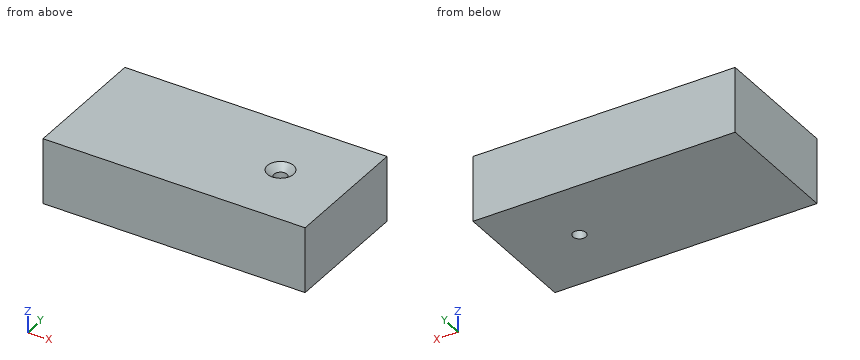
from build123d import *

# Parameters (mm, degrees)
F0_W           = 200
F0_H           = 100
F1_DEPTH       = 50
F3_D           = 10
F3_CSINK_D     = 20
F3_CSINK_ANGLE = 90


with BuildPart() as f1:
    # F0 (on Top) → F1 (new body)
    with BuildSketch(Plane.XY):
        with Locations((100, 50)):
            Rectangle(F0_W, F0_H)
    extrude(amount=F1_DEPTH)

    # F3 (through all)
    with Locations(Plane.XY.offset(50)):
        with Locations((150, 50)):
            CounterSinkHole(F3_D / 2, F3_CSINK_D / 2, counter_sink_angle=F3_CSINK_ANGLE)


solid = f1.part
Geometry: final body of the model. Coordinates: model frame, mm. Give positions to 0.01 mm unless a question says otherwise; leave off trailing zeros. Write each loop counter-clockwise with the first axis right and the second up, starting at its lowest first coordinate (ties: lowest second). Pieces come first, ordered by that corner, then holes. Notation, with made-up numbers: (-7.5, 84.25) -> (38.5, 84.25) arc R17 ccw to (38.5, 107.25) -> close; hole circle Ø6 at (72.25, 15.5). An arc over 180 degrees is marked (long way). Answer as a JSON object with one key per item and string values.
1. Cut plane A-A on x = 150. Output: boundary loops of the cut face in (y, z), and give its area (4 significant figures).
Ans:
{"outline": "(0, 0) -> (45, 0) -> (45, 45) -> (40, 50) -> (0, 50) -> close; (55, 0) -> (100, 0) -> (100, 50) -> (60, 50) -> (55, 45) -> close", "area": "4,475 mm^2"}
2. Ray query, probe 1 along X at (y, z) = (50, 10); probe 2 along Y at (x, z) = (150, 17); probe 3 along Z at (x, y) = (142.5, 44). Return the intervals inside material, ascending. Write a range as from..to.
Ans:
{"probe 1": "x = 0..145, 155..200", "probe 2": "y = 0..45, 55..100", "probe 3": "z = 0..49.6"}
3. Cut plane B-B on y = 50. Output: boundary loops of the cut face in (x, z).
Ans:
{"outline": "(0, 0) -> (145, 0) -> (145, 45) -> (140, 50) -> (0, 50) -> close; (155, 0) -> (200, 0) -> (200, 50) -> (160, 50) -> (155, 45) -> close"}
4. Contact query for a flat-ended pin moving along its axis: pin 1 (6 mm diameter, centred on x = 150, y = 50, fed in from -Z). Output: stop coordinate, or through.
Ans:
{"pin 1": "passes through"}
